```python
from build123d import *

# Parameters (mm, degrees)
SKETCH1_W               = 77.928270256
SKETCH1_H               = 65
BOSS_EXTRUDE1_DEPTH     = 2
CUT_EXTRUDE3_DEPTH      = 51.778477983
CUT_EXTRUDE3_DEPTH_BACK = 51.778477983
SKETCH2_R               = 1.55
SKETCH2_R_2             = 1.6
FILLET1_R               = 3


with BuildPart() as part:
    # Sketch1 → Boss-Extrude1 (new body)
    with BuildSketch(Plane(origin=(0, 0, 0), x_dir=(1, 0, 0), z_dir=(0, 1, 0))):
        Rectangle(SKETCH1_W, SKETCH1_H)
    extrude(amount=BOSS_EXTRUDE1_DEPTH)

    # Sketch2 → Cut-Extrude3 (cut, two sides: drawn at the far end of the back side and taken through both)
    with BuildSketch(Plane(origin=(0, 2, 0), x_dir=(1, 0, 0), z_dir=(0, 1, 0)).offset(-CUT_EXTRUDE3_DEPTH_BACK)):
        with Locations(Location((-24, 18, 0), (0, 0, 270))):
            Circle(SKETCH2_R)
        with Locations(Location((24, 18, 0), (0, 0, 270))):
            Circle(SKETCH2_R)
        with Locations(Location((24, -18, 0), (0, 0, 270))):
            Circle(SKETCH2_R)
        with Locations(Location((-24, -18, 0), (0, 0, 270))):
            Circle(SKETCH2_R)
        with Locations(Location((-11.865042966, 8.887432286, 0), (0, 0, 270))):
            Circle(SKETCH2_R_2)
        with Locations(Location((12.134957034, 8.887432286, 0), (0, 0, 270))):
            Circle(SKETCH2_R_2)
        with Locations(Location((12.134957034, -9.112567714, 0), (0, 0, 270))):
            Circle(SKETCH2_R_2)
        with Locations(Location((-11.865042966, -9.112567714, 0), (0, 0, 270))):
            Circle(SKETCH2_R_2)
    extrude(amount=CUT_EXTRUDE3_DEPTH + CUT_EXTRUDE3_DEPTH_BACK, mode=Mode.SUBTRACT)

    # Fillet1
    fillet1_edges = [part.edges().sort_by_distance(p)[0] for p in [
        (-38.964135128, 1, 32.5),
        (38.964135128, 1, 32.5),
        (38.964135128, 1, -32.5),
        (-38.964135128, 1, -32.5),
    ]]
    fillet(fillet1_edges, radius=FILLET1_R)


solid = part.part
```
Geometry: final body of the model. Coordinates: model frame, mm. Round coordinates to 2 decimals unless told otherwise and drop trailing zeros. Write each loop counter-clockwise with the first axis right and the second up, starting at its lowest first coordinate (ties: lowest second). Pieces come first, ordered by that corner, then holes.
Item 1: Mould query, pull axis Z, two halves, no side actions, for faces 1 (the face through (13.484, 0.986, -8.027)), 2 (the face through (-1, 1, -32.5)), 3 (the face through (13.484, 0.986, 9.973)), 4 (the face through (-38.109, 1.014, 31.598)). Classes: +Z half, -Z half, draft (parallel to the pull), parting line (faces both ways), or undercut.
Item 2: Section query A-A (z = 18). Return loops of the section in (x, y), plus the area to 3 significant figures.
Item 3: Section query B-B (x = 24). Return loops of the section in (y, z), plus the area to 3 significant figures.
Item 4: Material intervals for L1, parallel to X at y = 1.6, z = -18; L2, parallel to Z at x = 13, y = 0.6; L3, parallel to Z at x = -23.5, y = 1.5, sorted ascending.
Completed:
1. face 1: undercut
1. face 2: -Z half
1. face 3: undercut
1. face 4: +Z half
2. outline: (-38.96, 0) - (-25.55, 0) - (-25.55, 2) - (-38.96, 2) - close; (-22.45, 0) - (22.45, 0) - (22.45, 2) - (-22.45, 2) - close; (25.55, 0) - (38.96, 0) - (38.96, 2) - (25.55, 2) - close
2. area: 143 mm2
3. outline: (0, -32.5) - (2, -32.5) - (2, -19.55) - (0, -19.55) - close; (0, -16.45) - (2, -16.45) - (2, 16.45) - (0, 16.45) - close; (0, 19.55) - (2, 19.55) - (2, 32.5) - (0, 32.5) - close
3. area: 118 mm2
4. L1: x = -38.96 to -25.55, -22.45 to 22.45, 25.55 to 38.96
4. L2: z = -32.5 to -10.23, -7.54 to 7.77, 10.46 to 32.5
4. L3: z = -32.5 to -19.47, -16.53 to 16.53, 19.47 to 32.5
